Design review of the part built by this model. Coordinates are the model's own, in mm. A direction names the side the tool comes from. Give positions to 0.01 mm unless a question says otherwise; leave off trailing zeros. Write each loop counter-clockwise with the first axis right and the second up, starting at its lowest first coordinate (ties: lowest second). Pieces come first, ordered by that corner, then holes. Notation, with made-up numbers: M 38,14.5 L 73,14.5 A27 ccw 73,48.5 Z; hole C 41,43.25 d1. An arc over 180 degrees is marked long. One line per item, written item: value. Start each with the question number.
```python
from build123d import *

# Parameters (mm, degrees)
SKETCH1_R                   = 18.288
BOSS_EXTRUDE1_DEPTH         = 19.05
SKETCH3_R                   = 13.208
CUT_EXTRUDE1_DEPTH          = 33.121712096
SKETCH15_W                  = 19.05
SKETCH15_H                  = 17.526
BOSS_EXTRUDE3_DEPTH         = 15.24
SKETCH16_W                  = 11.43
SKETCH16_H                  = 5.842
CUT_EXTRUDE4_DEPTH          = 39.82462909
CHAMFER1_SIZE               = 8.129699408
CHAMFER1_SIZE_2             = 5.08
F_1_4_CLEARANCE_HOLE1_D     = 6.7564
F_1_4_CLEARANCE_HOLE1_DEPTH = 3.448428068
SKETCH19_R                  = 18.288
SKETCH19_R_2                = 13.208
CUT_EXTRUDE5_DEPTH          = 0.762
CUT_EXTRUDE6_START          = -2.54
SKETCH20_R                  = 18.288
CUT_EXTRUDE6_DEPTH          = 2.54
SKETCH21_R                  = 18.288
CUT_EXTRUDE7_DEPTH          = 7.493
SKETCH22_W                  = 19.05
SKETCH22_H                  = 4.191
CUT_EXTRUDE8_DEPTH          = 42.148
SKETCH24_R                  = 14.478
CUT_EXTRUDE10_DEPTH         = 5.334
SKETCH25_W                  = 8.255
SKETCH25_H                  = 5.08
BOSS_EXTRUDE4_DEPTH         = 15.24
F_4_CLEARANCE_HOLE1_D       = 3.4544
SKETCH28_W                  = 6.858
SKETCH28_H                  = 2.794
CUT_EXTRUDE11_DEPTH         = 43.003222079
MIRROR3_COPY_1_SKETCH_W     = 6.858
MIRROR3_COPY_1_SKETCH_H     = 2.794
MIRROR3_COPY_1_DEPTH        = 43.003222079
SKETCH30_W                  = 69.645379109
SKETCH30_H                  = 31.008453513
CUT_EXTRUDE13_DEPTH         = 24.638
CHAMFER2_SIZE               = 1.27


# Some blends are built 0.0001 mm under size
with BuildPart() as part:
    # Sketch1 → Boss-Extrude1 (new body)
    with BuildSketch(Plane.XY):
        with Locations(Location((0, 0, 0), (0, 0, 180))):
            Circle(SKETCH1_R)
    extrude(amount=BOSS_EXTRUDE1_DEPTH)

    # Sketch3 → Cut-Extrude1 (cut, through all)
    with BuildSketch(Plane.XY.offset(19.05)):
        Circle(SKETCH3_R)
    extrude(amount=-CUT_EXTRUDE1_DEPTH, mode=Mode.SUBTRACT)

    # Sketch15 → Boss-Extrude3 (add)
    with BuildSketch(Plane(origin=(0, -13.716, 0), x_dir=(1, 0, 0), z_dir=(0, 1, 0))):
        with Locations((0, -9.525)):
            Rectangle(SKETCH15_W, SKETCH15_H)
    extrude(amount=-BOSS_EXTRUDE3_DEPTH)

    # Sketch16 → Cut-Extrude4 (cut, through all)
    with BuildSketch(Plane.XY.offset(18.288)):
        with Locations((0, -22.586571932)):
            Rectangle(SKETCH16_W, SKETCH16_H)
    extrude(amount=-CUT_EXTRUDE4_DEPTH, mode=Mode.SUBTRACT)

    # Chamfer1
    # the kernel refuses this chamfer: 8.129699408, 5.08 mm, written as the material it takes off along each edge
    with BuildSketch(Plane(origin=(-30.543101737, -28.956, 0.762), x_dir=(0, 0.9997899140358644, -0.020497019104217945), z_dir=(1, 0, 0))) as chamfer1_piece_1:
        Polygon((CHAMFER1_SIZE * 0.999789913978, CHAMFER1_SIZE * 0.020497019103), (-CHAMFER1_SIZE_2 * 0.0204970191042, CHAMFER1_SIZE_2 * 0.999789914036), (0, 0), align=None)
    extrude(amount=61.086203475, mode=Mode.SUBTRACT)

    # 1/4 Clearance Hole1
    with Locations(Plane(origin=(0, -28.956, 0), x_dir=(-1, 0, 0), z_dir=(0, -1, 0))):
        with Locations((0, -12.021417661)):
            Hole(F_1_4_CLEARANCE_HOLE1_D / 2, depth=F_1_4_CLEARANCE_HOLE1_DEPTH)

    # Sketch19 → Cut-Extrude5 (cut)
    with BuildSketch(Plane.XY.offset(19.05)):
        with Locations(Location((0, 0, 0), (0, 0, 238.611833536))):
            Circle(SKETCH19_R)
        Circle(SKETCH19_R_2, mode=Mode.SUBTRACT)
    extrude(amount=-CUT_EXTRUDE5_DEPTH, mode=Mode.SUBTRACT)

    # Sketch20 → Cut-Extrude6 (cut)
    with BuildSketch(Plane.XY.offset(18.288).offset(CUT_EXTRUDE6_START)):
        with Locations(Location((0, 0, 0), (0, 0, 238.611833536))):
            Circle(SKETCH20_R)
    extrude(amount=CUT_EXTRUDE6_DEPTH, mode=Mode.SUBTRACT)

    # Sketch21 → Cut-Extrude7 (cut)
    with BuildSketch(Plane(origin=(0, 0, 0), x_dir=(-1, 0, 0), z_dir=(0, 0, -1))):
        Circle(SKETCH21_R)
    extrude(amount=-CUT_EXTRUDE7_DEPTH, mode=Mode.SUBTRACT)

    # Sketch22 → Cut-Extrude8 (cut, through all)
    with BuildSketch(Plane(origin=(0, -13.716, 0), x_dir=(1, 0, 0), z_dir=(0, 1, 0))):
        with Locations((0, -2.8575)):
            Rectangle(SKETCH22_W, SKETCH22_H)
    extrude(amount=-CUT_EXTRUDE8_DEPTH, mode=Mode.SUBTRACT)

    # Sketch24 → Cut-Extrude10 (cut)
    with BuildSketch(Plane.XY.offset(13.843)):
        Circle(SKETCH24_R)
    extrude(amount=-CUT_EXTRUDE10_DEPTH, mode=Mode.SUBTRACT)

    # Sketch25 → Boss-Extrude4 (add)
    with BuildSketch(Plane(origin=(13.208, 0, 0), x_dir=(0, 0, -1), z_dir=(1, 0, 0))):
        with Locations((-11.6205, 8.89)):
            Rectangle(SKETCH25_W, SKETCH25_H)
        with Locations((-11.6205, -8.89)):
            Rectangle(SKETCH25_W, SKETCH25_H)
    boss_extrude4 = extrude(amount=BOSS_EXTRUDE4_DEPTH)

    # #4 Clearance Hole1 (through all)
    with Locations(Plane(origin=(0, -11.43, 0), x_dir=(-1, 0, 0), z_dir=(0, -1, 0))):
        with Locations((-23.368, -11.6205)):
            f_4_clearance_hole1 = Hole(F_4_CLEARANCE_HOLE1_D / 2)

    # Sketch28 → Cut-Extrude11 (cut, through all)
    with BuildSketch(Plane.XY.offset(15.748)):
        with Locations((23.368, -8.89)):
            Rectangle(SKETCH28_W, SKETCH28_H)
    cut_extrude11 = extrude(amount=-CUT_EXTRUDE11_DEPTH, mode=Mode.SUBTRACT)

    # Mirror2: Cut-Extrude11 across plane
    add(cut_extrude11.mirror(Plane.ZX), mode=Mode.SUBTRACT)

    # Mirror3: Boss-Extrude4, #4 Clearance Hole1, Cut-Extrude11 across plane
    add(boss_extrude4.mirror(Plane(origin=(0, 0, 0), x_dir=(0, 0, 1), z_dir=(1, 0, 0))))
    add(f_4_clearance_hole1.mirror(Plane(origin=(0, 0, 0), x_dir=(0, 0, 1), z_dir=(1, 0, 0))), mode=Mode.SUBTRACT)
    add(cut_extrude11.mirror(Plane(origin=(0, 0, 0), x_dir=(0, 0, 1), z_dir=(1, 0, 0))), mode=Mode.SUBTRACT)

    # Mirror3 copy 1 sketch → Mirror3 copy 1 (cut, through all)
    with BuildSketch(Plane(origin=(0, 0, 15.748), x_dir=(-1, 0, 0), z_dir=(0, 0, 1))):
        with Locations((23.368, -8.89)):
            Rectangle(MIRROR3_COPY_1_SKETCH_W, MIRROR3_COPY_1_SKETCH_H)
    extrude(amount=-MIRROR3_COPY_1_DEPTH, mode=Mode.SUBTRACT)

    # Sketch30 → Cut-Extrude13 (cut)
    with BuildSketch(Plane(origin=(0, 18.288, 0), x_dir=(1, 0, 0), z_dir=(0, 1, 0))):
        with Locations((0.103127413, -15.504226757)):
            Rectangle(SKETCH30_W, SKETCH30_H)
    extrude(amount=-CUT_EXTRUDE13_DEPTH, mode=Mode.SUBTRACT)

    # Chamfer2
    chamfer2_edges = [part.edges().sort_by_distance(p)[0] for p in [
        (0, -14.478, 13.843),
        (0, -14.478, 8.509),
    ]]
    chamfer(chamfer2_edges, length=CHAMFER2_SIZE - 0.0001)  # a hair under: the kernel refuses the full size


solid = part.part
```
Q1. The part is to be moulded in two halves that separate along Z. For faces 1 (the face through (-5.715, -23, 12)), 2 (the face through (-0.2, -13.4, 8.7)), 3 (the face through (0, -19, 4.953)), say which applies: pulls with the +Z half, pulls with the -Z half, needs draft (parallel to the pull), parting line crosses it, or undercut.
Q2. Take a section at A-A, the plane y = -21.75. Give the boundary of the cut face in (x, z) (3 decimals), then the cut area to 3 significant figures.
Q3. Take a section at B-B, the plane y = -8.5. State how many separate pieces and enclosed holes the cut face has, then the cut area to 3 significant figures.
Q4. Wall thickness on line 1 (Y direction, x = -24.5, z = 8.25); line 2 (X direction, y = -10, z = 14); line 3 (X direction, y = -22, z = 9) (3 decimals): over which ranges is each line inside the solid? List them lowest first. Write a range as from..to.
Q5. For P1, Ø10, axis at x = -13, y = -9, coming from the +Z side; P2, Ø5, axis at x = 4.5, y = -13, coming from the -Z side; P3, Ø6, axis at x = 0, z = 12.02, coming from the +Y side, all flat-tipped, find the tip position at first contact; note any pin that passes through.
Q6. Machinability: for faces 4 (the face through (0.14, -18.287, 6.205)), 5 (the face through (-0.14, -18.287, 17)), 6 (the face through (-22, -7.493, 13)), 7 (the face through (-0.44, -27.21, 8.67)), which of the approach directions +Z, -Z, +X, -X, +Y, -Y give a long, thin tool a straight path to every point of the face, cutting with its end or side? Answer none if there is none.
Results list:
1. face 1: needs draft
1. face 2: undercut
1. face 3: pulls with the -Z half
2. outline: M -9.525,4.953 L -5.715,4.953 L -5.715,18.288 L -9.525,18.288 Z; M 5.715,4.953 L 9.525,4.953 L 9.525,18.288 L 5.715,18.288 Z
2. area: 102 mm^2
3. separate pieces: 4
3. enclosed holes: 0
3. area: 176 mm^2
4. line 1: y = -11.43..-10.29, -7.49..-6.35
4. line 2: x = -28.45..-26.8, -19.94..-8.63, 8.63..19.94, 26.8..28.45
4. line 3: x = -9.525..-5.715, 5.715..9.525
5. P1: stops at z = 15.75
5. P2: stops at z = 7.49
5. P3: stops at y = -12.99
6. face 4: -Z, +Y
6. face 5: +Z, +Y
6. face 6: +Z, -Z
6. face 7: -Y
